For this review, take the finished solid that the model builds, in its own axes (mm). Round coordinates to 2 decimals unless told otherwise and drop trailing zeros. Loops run counter-clockwise (first coordinate to the right, second up) from the corner with the lowest first, then second, coordinate; pieces in that order, holes last. Notation, with made-up numbers: M 66.25,82 L 93.25,82 A18 ccw 93.25,115 Z; hole C 51.25,-22 d3. An arc over 180 degrees is marked long. Write item = value, one per line. Start each with the question number.
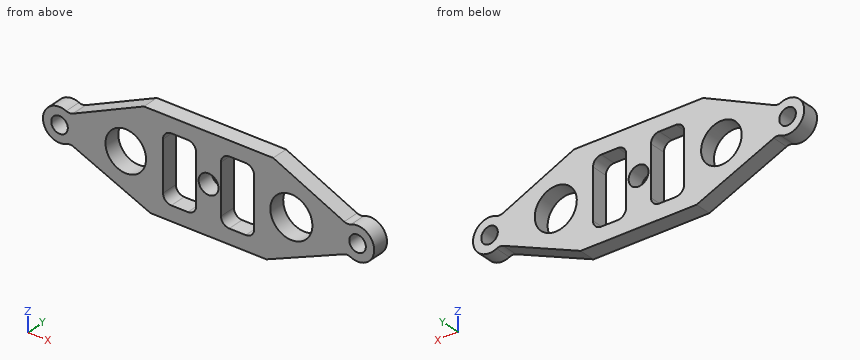
```python
from build123d import *

# Parameters (mm, degrees)
CROQUIS1_R              = 12.7
CROQUIS1_R_2            = 12.25
CROQUIS1_R_3            = 5
CROQUIS1_R_4            = 6
SALIENTE_EXTRUIR1_DEPTH = 10


with BuildPart() as part:
    # Croquis1 → Saliente-Extruir1 (new body)
    with BuildSketch(Plane(origin=(0, 0, 0), x_dir=(1, 0, 0), z_dir=(0, 1, 0))):
        with BuildLine():
            Line((-35, 28.891912333), (35, 28.891912333))
            Line((35, 28.891912333), (81.677313088, 8.985147888))
            ThreePointArc((81.677313088, 8.985147888), (83.725830982, 8.585112915), (85.759177009, 9.056236545))
            ThreePointArc((85.759177009, 9.056236545), (99.999086859, 0.13513694), (86.005469996, -9.167536749))
            ThreePointArc((86.005469996, -9.167536749), (83.960134549, -8.751536206), (81.923175769, -9.206786103))
            Line((81.923175769, -9.206786103), (39.017575448, -28.891912333))
            Line((39.017575448, -28.891912333), (-39.017575448, -28.891912333))
            Line((-39.017575448, -28.891912333), (-81.923175769, -9.206786103))
            ThreePointArc((-81.923175769, -9.206786103), (-83.960134549, -8.751536206), (-86.005469996, -9.167536749))
            ThreePointArc((-86.005469996, -9.167536749), (-99.999086859, 0.13513694), (-85.759177009, 9.056236545))
            ThreePointArc((-85.759177009, 9.056236545), (-83.725830982, 8.585112915), (-81.677313088, 8.985147888))
            Line((-81.677313088, 8.985147888), (-35, 28.891912333))
        make_face()
        with Locations(Location((50, 0, 0), (0, 0, 270))):
            Circle(CROQUIS1_R, mode=Mode.SUBTRACT)
        with Locations(Location((-50, 0, 0), (0, 0, 270))):
            Circle(CROQUIS1_R_2, mode=Mode.SUBTRACT)
        with Locations(Location((-90, 0, 0), (0, 0, 270))):
            Circle(CROQUIS1_R_3, mode=Mode.SUBTRACT)
        with Locations(Location((90, 0, 0), (0, 0, 270))):
            Circle(CROQUIS1_R_3, mode=Mode.SUBTRACT)
        with Locations(Location((0, 0, 0), (0, 0, 270))):
            Circle(CROQUIS1_R_4, mode=Mode.SUBTRACT)
        with BuildLine():
            Line((-22.5, 20), (-12.5, 20))
            ThreePointArc((-12.5, 20), (-8.964466094, 18.535533906), (-7.5, 15))
            Line((-7.5, 15), (-7.5, -15))
            ThreePointArc((-7.5, -15), (-8.964466094, -18.535533906), (-12.5, -20))
            Line((-12.5, -20), (-22.5, -20))
            ThreePointArc((-22.5, -20), (-26.035533906, -18.535533906), (-27.5, -15))
            Line((-27.5, -15), (-27.5, 15))
            ThreePointArc((-27.5, 15), (-26.035533906, 18.535533906), (-22.5, 20))
        make_face(mode=Mode.SUBTRACT)
        with BuildLine():
            Line((12.5, 20), (22.5, 20))
            ThreePointArc((22.5, 20), (26.035533906, 18.535533906), (27.5, 15))
            Line((27.5, 15), (27.5, -15))
            ThreePointArc((27.5, -15), (26.035533906, -18.535533906), (22.5, -20))
            Line((22.5, -20), (12.5, -20))
            ThreePointArc((12.5, -20), (8.964466094, -18.535533906), (7.5, -15))
            Line((7.5, -15), (7.5, 15))
            ThreePointArc((7.5, 15), (8.964466094, 18.535533906), (12.5, 20))
        make_face(mode=Mode.SUBTRACT)
    extrude(amount=SALIENTE_EXTRUIR1_DEPTH)


solid = part.part
```
(1) Add section A-A on x = 0. Write out the cut boundary in (y, z).
(2) Add section B-B on z = 0. Count the separate pieces of the cut face and the enclosed holes in it, and give its area (3 significant figures).
(3) Wall thickness on L1, parallel to Z at x = 16.5, y = 8; L2, parallel to X at y = 8.5, z = 19.5; L3, parallel to X at y = 5.75, z = -16: over which ranges is each line inside the solid? List them lowest first.
(4) Add section D-D on x = -90. Write out the cut boundary in (y, z), and give its area (3 significant figures).
(5) For pin 1 Ø1.5 at (y, z) = (8.5, 22.5) entering from +X; pin 2 Ø1.5 at (x, y) = (74.5, 1) entering from +Z; pin 3 Ø1.5 at (y, z) = (7.5, 8.5) entering from +X; pin 4 Ø7 at (x, z) = (0, 0) entering from -Y, all flat-tipped, find the tip position at first contact; note any pin that passes through.
Answer sheet:
q1.outline = M 0,-28.89 L 10,-28.89 L 10,-6 L 0,-6 Z; M 0,6 L 10,6 L 10,28.89 L 0,28.89 Z
q2.separate_pieces = 8
q2.enclosed_holes = 0
q2.area = 781 mm²
q3.L1 = -28.89 to -20, 20 to 28.89
q3.L2 = -59.49 to -24.68, -10.32 to 10.32, 24.68 to 59.49
q3.L3 = -65.23 to -27.4, -7.6 to 7.6, 27.4 to 65.23
q4.outline = M 0,-10 L 10,-10 L 10,-5 L 0,-5 Z; M 0,5 L 10,5 L 10,10 L 0,10 Z
q4.area = 100 mm²
q5.pin_1 = 54.58
q5.pin_2 = 12.96
q5.pin_3 = 96.32
q5.pin_4 = through
